```python
from build123d import *

# Parameters (mm, degrees)
SKETCH1_W                                        = 75
SKETCH1_H                                        = 90
BOSS_EXTRUDE1_DEPTH                              = 22
CBORE_FOR_M10_SOCKET_HEAD_CAP_SCREW1_D           = 12
CBORE_FOR_M10_SOCKET_HEAD_CAP_SCREW1_CBORE_D     = 18
CBORE_FOR_M10_SOCKET_HEAD_CAP_SCREW1_CBORE_DEPTH = 31
CHAMFER1_SIZE                                    = 5


with BuildPart() as part:
    # Sketch1 → Boss-Extrude1 (new body)
    with BuildSketch(Plane.XY):
        with Locations((0, 45)):
            Rectangle(SKETCH1_W, SKETCH1_H)
    extrude(amount=BOSS_EXTRUDE1_DEPTH)

    # CBORE for M10 Socket Head Cap Screw1 (through all)
    with Locations(Plane(origin=(0, 90, 0), x_dir=(-1, 0, 0), z_dir=(0, 1, 0))):
        with Locations((25, 11), (-25, 11)):
            CounterBoreHole(CBORE_FOR_M10_SOCKET_HEAD_CAP_SCREW1_D / 2, CBORE_FOR_M10_SOCKET_HEAD_CAP_SCREW1_CBORE_D / 2, CBORE_FOR_M10_SOCKET_HEAD_CAP_SCREW1_CBORE_DEPTH)

    # Chamfer1
    # the kernel refuses this chamfer: 5 mm, written as the material it takes off along each edge
    with BuildSketch(Plane(origin=(-37.5, 90, -12.85841494), x_dir=(-0.027495876610586282, -0.9996219169112968, 0), z_dir=(0, 0, 1))) as chamfer1_piece_1:
        Polygon((CHAMFER1_SIZE * 0.999621916911, CHAMFER1_SIZE * 0.0274958766106), (-CHAMFER1_SIZE * 0.0274958766106, CHAMFER1_SIZE * 0.999621916911), (0, 0), align=None)
    extrude(amount=47.71682988, mode=Mode.SUBTRACT)
    with BuildSketch(Plane(origin=(37.5, 90, -12.85841494), x_dir=(0.027495876610586282, -0.9996219169112968, 0), z_dir=(0, 0, 1))) as chamfer1_piece_2:
        Polygon((CHAMFER1_SIZE * 0.999621916911, -CHAMFER1_SIZE * 0.0274958766106), (-CHAMFER1_SIZE * 0.0274958766106, -CHAMFER1_SIZE * 0.999621916911), (0, 0), align=None)
    extrude(amount=47.71682988, mode=Mode.SUBTRACT)


solid = part.part
```
Source: CAD feature listing. Evaluate the final solid. Frame: model axes, mm. A direction names the side the tool comes from. Coordinates: 2 decimals unless noted, no trailing zeros. Loops run counter-clockwise (first coordinate to the right, second up) from the corner with the lowest first, then second, coordinate; pieces in that order, holes last. Notation, with made-up numbers: M 45.25,-35.75 L 81.25,-35.75 A26 ccw 81.25,-13.75 Z; hole C 63.25,46.5 d10. An arc over 180 degrees is marked long. Use CSV: the item, a comma, the result in double quotes.
(1) Contact query for flat-ended pins moving along their axis: pin 1 (12 mm diameter, centred on x = 28, z = 17.5, fed in from -Y); pin 2 (1.5 mm diameter, centred on x = 20.5, z = 8, fed in from +Y); pin 3 (5.5 mm diameter, centred on x = -25, z = 13.5, fed in from +Y). Output: stop coordinate, or through.
Answers follow:
pin 1,"y = 0"
pin 2,"y = 59"
pin 3,"through"
(2) Cut plane A-A on z = 11. Return loops of the section in (x, y), and give its area (3 significant figures).
Answers follow:
outline,"M -37.5,0 L -31,0 L -31,59 L -34,59 L -34,88.5 L -37.5,85 Z; M -19,0 L 19,0 L 19,59 L 16,59 L 16,90 L -16,90 L -16,59 L -19,59 Z; M 31,0 L 37.5,0 L 37.5,85 L 34,88.5 L 34,59 L 31,59 Z"
area,"4,200 mm²"
(3) Line query: line 1 (X direction, y = 70.5, z = 11); line 2 (Z direction, x = -25, y = 13); line 3 (X direction, y = 62, z = 7.25). Output: solid intervals per line, ascending. Write a range as [from, to].
Answers follow:
line 1,"[-37.5, -34], [-16, 16], [34, 37.5]"
line 2,"[0, 5], [17, 22]"
line 3,"[-37.5, -33.18], [-16.82, 16.82], [33.18, 37.5]"
(4) Draft query along X for faces 3 (the face through (20.24, 29.09, 7.35)), 4 (the face through (16.686, 74.717, 7.553)), 5 (the face through (-1, 46, 0)), 6 (the face through (37.5, 42, 11)). Return one class per face: pulls with the +X half, pulls with the -X half, needs draft (parallel to the pull), parting line crosses it, or undercut.
Answers follow:
face 3,"undercut"
face 4,"undercut"
face 5,"needs draft"
face 6,"pulls with the +X half"
(5) Cut plane C-C on y = 76.5. Return loops of the section in (x, z).
Answers follow:
outline,"M -37.5,0 L 37.5,0 L 37.5,22 L -37.5,22 Z; hole C -25,11 d18; hole C 25,11 d18"
(6) Cut plane B-B on x = 25. Return loops of the section in (y, z), and give its area (3 significant figures).
Answers follow:
outline,"M 0,0 L 90,0 L 90,2 L 59,2 L 59,5 L 0,5 Z; M 0,17 L 59,17 L 59,20 L 90,20 L 90,22 L 0,22 Z"
area,"714 mm²"
(7) Cut plane D-D on z = 4. Return loops of the section in (x, y).
Answers follow:
outline,"M -37.5,0 L 37.5,0 L 37.5,85 L 32.5,90 L 30.66,90 L 30.66,59 L 19.34,59 L 19.34,90 L -19.34,90 L -19.34,59 L -30.66,59 L -30.66,90 L -32.5,90 L -37.5,85 Z"
(8) Reachability of faces 1 (the face through (-35, 87.5, 10.8)), 2 (the face through (-33.314, 74.717, 7.553)) from +Z, -Z, +X, -X, +Y, -Y: full face, straight path, thin tool, end or side. Return the list, or none.
Answers follow:
face 1,"+Z, -Z, -X, +Y"
face 2,"+Y"
